The drawing under review shows one solid part. Ordinate dimensions are in mm from its lowest x, y, z. A direction names the side the tool comes from. Coordinates: 2 decimals unless noted, no trailing zeros. Loops run counter-clockwise (first coordinate to the right, second up) from the corner with the lowest first, then second, coordinate; pieces in that order, holes last. Notation, with made-up numbers: M 63,57 L 69,57 A12 cw 69,63 Z; hole C 53,60 d7. An arc over 180 degrees is marked long. Return JSON: item names as keys, results as strings.
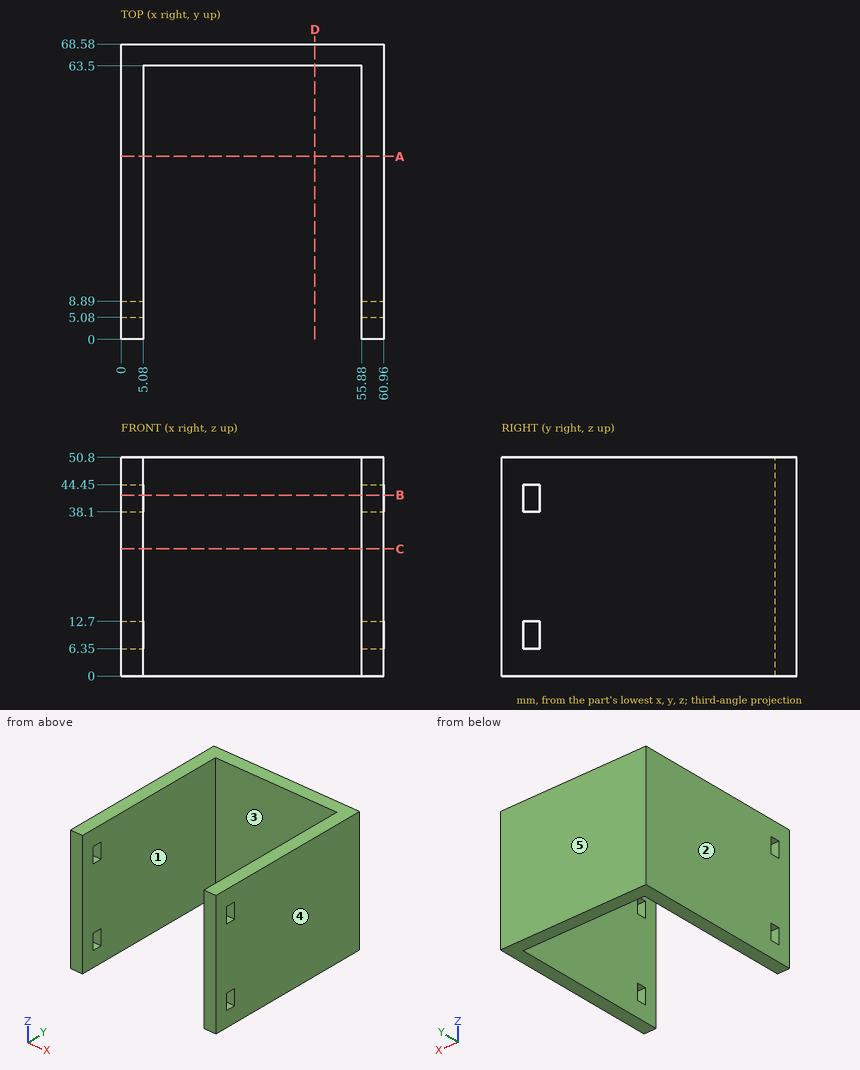
1. Add section C-C on z = 29.5. Give the boundary of the cut face in (x, y), plus the area to 3 significant figures.
Check values:
{"outline": "M 0,0 L 5.08,0 L 5.08,63.5 L 55.88,63.5 L 55.88,0 L 60.96,0 L 60.96,68.58 L 0,68.58 Z", "area": "955 mm²"}
2. To check wall thickness, follow line 1 (X direction, y = 16, z = 42.5); line 2 (Y direction, x = 52, z = 5.5). State the ranges of each line that lie inside material, in increasing order.
Check values:
{"line 1": "0 to 5.08, 55.88 to 60.96", "line 2": "63.5 to 68.58"}
3. Add section D-D on x = 45. Give the boundary of the cut face in (y, z), plus the area to 3 significant figures.
Check values:
{"outline": "M 63.5,0 L 68.58,0 L 68.58,50.8 L 63.5,50.8 Z", "area": "258 mm²"}
4. The part is to be moulded in two halves that separate along X. For the marked faces 3, 4 and 5, say which applies: released by +X, released by -X, zero draft, split by the parting line, or undercut.
Check values:
{"face 3": "undercut", "face 4": "released by +X", "face 5": "zero draft"}
5. Machinability: for the marked faces 1 and 2, which of the approach directions +Z, -Z, +X, -X, +Y, -Y give a long, thin tool a straight path to every point of the face, cutting with its end or side? Answer none if there is none.
Check values:
{"face 1": "+Z, -Z, -Y", "face 2": "+Z, -Z, -X, +Y, -Y"}
6. Add section A-A on y = 42.5. Give the boundary of the cut face in (x, z).
Check values:
{"outline": "M 0,0 L 5.08,0 L 5.08,50.8 L 0,50.8 Z; M 55.88,0 L 60.96,0 L 60.96,50.8 L 55.88,50.8 Z"}
7. Add section B-B on z = 42. Give the boundary of the cut face in (x, y), plus the area to 3 significant figures.
Check values:
{"outline": "M 0,0 L 5.08,0 L 5.08,5.08 L 0,5.08 Z; M 0,8.89 L 5.08,8.89 L 5.08,63.5 L 55.88,63.5 L 55.88,8.89 L 60.96,8.89 L 60.96,68.58 L 0,68.58 Z; M 55.88,0 L 60.96,0 L 60.96,5.08 L 55.88,5.08 Z", "area": "916 mm²"}
